The listing builds one solid part. Answer for the finished solid, in the listing's coordinates (mm). Face numbers are marked on the shaded views. A direction names the side the tool comes from. Coordinates: 2 decimals unless noted, no trailing zeros. Order: outer loops, then holes, each group sorted by start corner. A loop starts at its lowest first (then second) coordinate and runs counter-clockwise, first axis right, second up. Notation, with made-up numbers: M -13.75,41.25 L 27.25,41.25 A29 ccw 27.25,69.25 Z; hole C -12.5,49 d9. An arc over 180 degrees is marked long. One line per item, written item: value. Start each with the question number.
Q1. The part is cut by section B-B on y = -7. Give the vertices of the cut face in (x, z), then the cut area to 3 significant figures.
Q2. The part is cut by section A-A on x = -33.5. Give the vertices of the cut face in (y, z), then the cut area to 3 significant figures.
Q3. The part is cut by section C-C on z = -1.75. Give the vertices of the cut face in (x, y), then the cut area to 3 significant figures.
Q4. The part is cut by section D-D on y = -9.75. Give the vertices of the cut face in (x, z), then the cut area to 3 significant figures.
Q5. Each of these flat-tipped pins is pushed along its axis until it touches: pin 1 Ø8 at (x, y) = (-1.5, -10.5) entering from +Z; pin 2 Ø1.5 at (y, z) = (-5, -1) entering from +X; pin 3 Ø1.5 at (x, y) = (-5.5, -6.5) entering from +Z. Where does it stop, or does it pass through?
Q6. Straight lines are drawn through the part: line 1 along Z through (x, y) = (-41, -0.75); line 2 along Y through (x, z) = (5.5, 2.5); line 3 along X through (y, z) = (-3.25, 1.5). For each, find the intervals that lie inside material, in ascending order. Write a range as [from, to].
Q7. For the marked faces 1 and 2, determine the directions among +Z, -Z, +X, -X, +Y, -Y from which every point of the face is accessible in a straight line to the end or side of a thin tool.
```python
from build123d import *

# Parameters (mm, degrees)
F1_DEPTH = 16
F3_DEPTH = 25
F4_R     = 4


with BuildPart() as f1:
    # F0 (on Front) → F1 (new body)
    with BuildSketch(Plane.XZ):
        Polygon((9.1923881554, 9.1923881554), (0, 0), (-50, 0), (-50, -3), (1.2426406871, -3), (11.313708499, 7.0710678119), align=None)
    extrude(amount=F1_DEPTH)

    # F2 (on face) → F3 (cut)
    with BuildSketch(Plane(origin=(0, 0, 0), x_dir=(0, -1, 0), z_dir=(-0.7071067812, 0, 0.7071067812))):
        with BuildLine():
            Line((5.1715728753, 10), (10.8284271247, 10))
            ThreePointArc((10.8284271247, 10), (8, 11), (5.1715728753, 10))
        make_face()
        with BuildLine():
            ThreePointArc((5.1715728753, 10), (6.0606601718, 2.4393398282), (12.5, 6.5))
            ThreePointArc((12.5, 6.5), (12.0606601718, 8.4393398282), (10.8284271247, 10))
            Line((10.8284271247, 10), (5.1715728753, 10))
        make_face()
        with BuildLine():
            ThreePointArc((5.1715728753, 10), (8, 11), (10.8284271247, 10))
            Line((10.8284271247, 10), (16, 10))
            Line((16, 10), (16, 13))
            Line((16, 13), (0, 13))
            Line((0, 13), (0, 10))
            Line((0, 10), (5.1715728753, 10))
        make_face()
    extrude(amount=-F3_DEPTH, mode=Mode.SUBTRACT)

    # F4
    f4_edges = [f1.edges().sort_by_distance(p)[0] for p in [
        (0, -8, 0),
    ]]
    fillet(f4_edges, radius=F4_R)


solid = f1.part
```
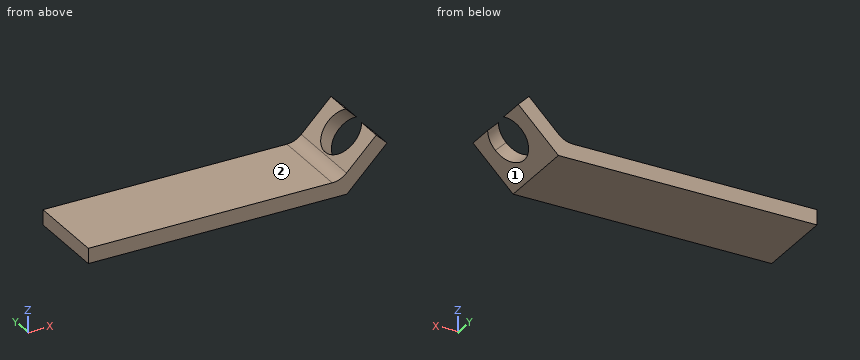
Output:
1. outline: M -50,-3 L 1.24,-3 L 3.62,-0.63 L 1.49,1.49 L 1.17,1.17 A4 cw -1.66,0 L -50,0 Z
1. area: 160 mm^2
2. outline: M -16,-3 L 0,-3 L 0,0 L -16,0 Z
2. area: 48.0 mm^2
3. outline: M -50,-16 L 2.49,-16 L 2.49,0 L -50,0 Z
3. area: 840 mm^2
4. outline: M -50,-3 L 1.24,-3 L 3.79,-0.46 L 1.66,1.66 L 1.17,1.17 A4 cw -1.66,0 L -50,0 Z
4. area: 161 mm^2
5. pin 1: stops at z = 2.42
5. pin 2: stops at x = 3.99
5. pin 3: stops at z = 0
6. line 1: z = [-3, 0]
6. line 2: y = [-16, -12.42], [-3.58, 0]
6. line 3: x = [1.5, 5.74]
7. face 1: -Z, +X, +Y, -Y
7. face 2: +Z, -X, +Y, -Y
